Verification items for the finished model (mm, model axes). A direction names the side the tool comes from. Round coordinates to 2 decimals unless told otherwise and drop trailing zeros. Write each loop counter-clockwise with the first axis right and the second up, starting at its lowest first coordinate (ties: lowest second). Pieces come first, ordered by that corner, then holes. Notation, with made-up numbers: M 26.5,71.25 L 33.5,71.25 A29 cw 33.5,107.25 Z; hole C 42,68.5 d6. An arc over 180 degrees is marked long. Write each question's results on one line, items separated by ' | '.
from build123d import *

# Parameters (mm, degrees)
SKETCH1_R                        = 175
BOSS_EXTRUDE1_DEPTH              = 30
TAP_DRILL_FOR_M10X1_5_TAP1_D     = 8.5
TAP_DRILL_FOR_M10X1_5_TAP1_DEPTH = 20
TAP_DRILL_FOR_M10X1_5_TAP1_TIP   = 2.553657631
SKETCH7_R                        = 175
BOSS_EXTRUDE2_DEPTH              = 20
F_6_0_6_DIAMETER_HOLE1_D         = 6
TAP_DRILL_FOR_M7X1_0_TAP2_D      = 6
TAP_DRILL_FOR_M7X1_0_TAP2_DEPTH  = 20
TAP_DRILL_FOR_M7X1_0_TAP2_TIP    = 1.802581857


with BuildPart() as part:
    # Sketch1 → Boss-Extrude1 (new body)
    with BuildSketch(Plane(origin=(0, 0, 0), x_dir=(1, 0, 0), z_dir=(0, 1, 0))):
        Circle(SKETCH1_R)
    extrude(amount=BOSS_EXTRUDE1_DEPTH)

    # Tap Drill for M10x1.5 Tap1
    with Locations(Plane(origin=(0, 30, 0), x_dir=(1, 0, 0), z_dir=(0, 1, 0))):
        with Locations((-106.066017178, -106.066017178), (106.066017178, -106.066017178), (106.066017178, 106.066017178), (-106.066017178, 106.066017178)):
            Hole(TAP_DRILL_FOR_M10X1_5_TAP1_D / 2, depth=TAP_DRILL_FOR_M10X1_5_TAP1_DEPTH)
            with Locations((0, 0, -(TAP_DRILL_FOR_M10X1_5_TAP1_DEPTH + TAP_DRILL_FOR_M10X1_5_TAP1_TIP / 2))):  # 118° drill point
                Cone(0, TAP_DRILL_FOR_M10X1_5_TAP1_D / 2, TAP_DRILL_FOR_M10X1_5_TAP1_TIP, mode=Mode.SUBTRACT)

    # Sketch7 → Boss-Extrude2 (add)
    with BuildSketch(Plane.XZ):
        Circle(SKETCH7_R)
    extrude(amount=BOSS_EXTRUDE2_DEPTH)

    # 6.0 _6_ Diameter Hole1 (through all)
    with Locations(Plane(origin=(0, 30, 0), x_dir=(1, 0, 0), z_dir=(0, 1, 0))):
        with Locations((-137.5, 0), (0, -137.5), (137.5, 0), (0, 137.5)):
            Hole(F_6_0_6_DIAMETER_HOLE1_D / 2)

    # Tap Drill for M7x1.0 Tap2
    with Locations(Plane(origin=(0, -20, 0), x_dir=(-1, 0, 0), z_dir=(0, -1, 0))):
        with Locations((78.367338092, 0.001727747), (-0.067861908, -78.484272253), (-78.503061908, 0.001727747), (-0.067861908, 78.487727747)):
            Hole(TAP_DRILL_FOR_M7X1_0_TAP2_D / 2, depth=TAP_DRILL_FOR_M7X1_0_TAP2_DEPTH)
            with Locations((0, 0, -(TAP_DRILL_FOR_M7X1_0_TAP2_DEPTH + TAP_DRILL_FOR_M7X1_0_TAP2_TIP / 2))):  # 118° drill point
                Cone(0, TAP_DRILL_FOR_M7X1_0_TAP2_D / 2, TAP_DRILL_FOR_M7X1_0_TAP2_TIP, mode=Mode.SUBTRACT)


solid = part.part
1) Sectioned sample at A-A, the plane z = 30.5. Record the cut outline in (x, y), and give its area (3 significant figures).
Calculated:
outline: M -172.32,-20 L 172.32,-20 L 172.32,30 L -172.32,30 Z | area: 17,200 mm²
2) Access from +Z, -Z, +X, -X, +Y, -Y to the whole of each face (thin tool, end or side, straight path). Record for faces 1 (the cylindrical face through (-102.9, 19.9, -108.9)), 2 (the flat face through (-2, -20, 2)).
Calculated:
face 1: +Y | face 2: +Z, -Z, +X, -X, -Y
3) Sectioned sample at B-B, the plane x = -66. Record the cut outline in (y, z).
Calculated:
outline: M -20,-162.08 L 30,-162.08 L 30,162.08 L -20,162.08 Z
4) Depth check by flat-ended pin: P1, Ø5, axis at x = 0, z = -137.5, coming from the +Y side; P2, Ø5, axis at x = 0.07, z = 78.48, coming from the -Y side; P3, Ø5, axis at x = -106.07, z = -106.07, coming from the +Y side; P4, Ø5, axis at y = 2, z = 62, coming from the +X side. Enter the tip coordinate at first touch or a pass-through.
Calculated:
P1: passes through | P2: stops at y = 0.3 | P3: stops at y = 8.95 | P4: stops at x = 164.57
5) Draft check along Z on faces 3 (the cylindrical face through (-128.982, 5.35, 118.273)), 4 (the conical face through (-106.226, 7.89, 106.787)), 5 (the flat face through (-2, 30, -2)), 6 (the cylindrical face through (110.312, 19.86, -106.253)). Enter one of: pulls with the +Z half, pulls with the -Z half, needs draft (parallel to the pull), parting line crosses it, or undercut.
Calculated:
face 3: parting line crosses it | face 4: undercut | face 5: needs draft | face 6: undercut
6) Material ranges on line 1 (Z direction, x = 0, y = 2); line 2 (Z direction, x = 0, y = -4); line 3 (X direction, y = -2, z = -137), recorded low to high. Write a range as [from, to].
Calculated:
line 1: z = [-175, -140.5], [-134.5, 134.5], [140.5, 175] | line 2: z = [-175, -140.5], [-134.5, -81.49], [-75.49, 75.49], [81.48, 134.5], [140.5, 175] | line 3: x = [-108.89, -2.96], [2.96, 108.89]
